The model under review builds one solid part; all positions refer to its coordinate system, in mm. Face numbers are marked on the shaded views. A direction names the side the tool comes from. Give positions to 0.01 mm unless a question says otherwise; leave off trailing zeros. Write each loop counter-clockwise with the first axis right and the second up, starting at its lowest first coordinate (ties: lowest second). Pieces come first, ordered by that corner, then holes. Notation, with made-up numbers: M -21.5,30.5 L 17.5,30.5 A25 cw 17.5,58.5 Z; hole C 35.25,-17 d11. An arc over 180 degrees is marked long. Write item = value, one per line. Start each with the question number.
```python
from build123d import *

# Parameters (mm, degrees)
F3_DEPTH = 25.4
F4_DEPTH = 25.4


with BuildPart() as f1:
    # F0 (on Front) → F1 (revolve)
    with BuildSketch(Plane.XZ):
        with BuildLine():
            Line((-95.25, -6.372012), (-95.25, -12.722012))
            Line((-95.25, -12.722012), (88.9, -12.722012))
            Line((88.9, -12.722012), (88.9, -0.022012))
            Line((88.9, -0.022012), (0, -0.022012))
            ThreePointArc((0, -0.022012), (-5.990472, -3.916067), (-12.7, -6.372012))
            Line((-12.7, -6.372012), (-45.3898, -6.372012))
            ThreePointArc((-45.3898, -6.372012), (-47.67075, -5.047272), (-47.6504, -2.409612))
            Line((-47.6504, -2.409612), (-52.4002, -2.409612))
            ThreePointArc((-52.4002, -2.409612), (-54.839819, -3.877688), (-57.640804, -4.389037))
            Line((-57.640804, -4.389037), (-93.039957, -4.389037))
            ThreePointArc((-93.039957, -4.389037), (-92.897345, -6.771022), (-95.25, -6.372012))
        make_face()
    revolve(axis=Axis((-3.175, 0, -12.722012), (1, 0, 0)))

    # F2 (on Front) → F3 (cut)
    with BuildSketch(Plane.XZ):
        with BuildLine():
            ThreePointArc((-12.482816, -6.482415), (1.656656, -10.036727), (16.186922, -11.232215))
            Line((16.186922, -11.232215), (87.516984, -11.232215))
            Line((87.516984, -11.232215), (89.117184, -12.832415))
            Line((89.117184, -12.832415), (96.563645, 18.124769))
            Line((96.563645, 18.124769), (7.196714, 21.508439))
            Line((7.196714, 21.508439), (-12.482816, -6.482415))
        make_face()
        with BuildLine():
            Line((96.563645, -43.789599), (89.117184, -12.832415))
            Line((89.117184, -12.832415), (87.516984, -14.432615))
            Line((87.516984, -14.432615), (16.186922, -14.432615))
            ThreePointArc((16.186922, -14.432615), (1.656656, -15.628103), (-12.482816, -19.182415))
            Line((-12.482816, -19.182415), (7.196714, -47.173269))
            Line((7.196714, -47.173269), (96.563645, -43.789599))
        make_face()
    extrude(amount=-F3_DEPTH, mode=Mode.SUBTRACT)

    # F2 (on Front) → F4 (cut)
    with BuildSketch(Plane.XZ):
        with BuildLine():
            ThreePointArc((-12.482816, -6.482415), (1.656656, -10.036727), (16.186922, -11.232215))
            Line((16.186922, -11.232215), (87.516984, -11.232215))
            Line((87.516984, -11.232215), (89.117184, -12.832415))
            Line((89.117184, -12.832415), (96.563645, 18.124769))
            Line((96.563645, 18.124769), (7.196714, 21.508439))
            Line((7.196714, 21.508439), (-12.482816, -6.482415))
        make_face()
        with BuildLine():
            Line((96.563645, -43.789599), (89.117184, -12.832415))
            Line((89.117184, -12.832415), (87.516984, -14.432615))
            Line((87.516984, -14.432615), (16.186922, -14.432615))
            ThreePointArc((16.186922, -14.432615), (1.656656, -15.628103), (-12.482816, -19.182415))
            Line((-12.482816, -19.182415), (7.196714, -47.173269))
            Line((7.196714, -47.173269), (96.563645, -43.789599))
        make_face()
    extrude(amount=F4_DEPTH, mode=Mode.SUBTRACT)


solid = f1.part
```
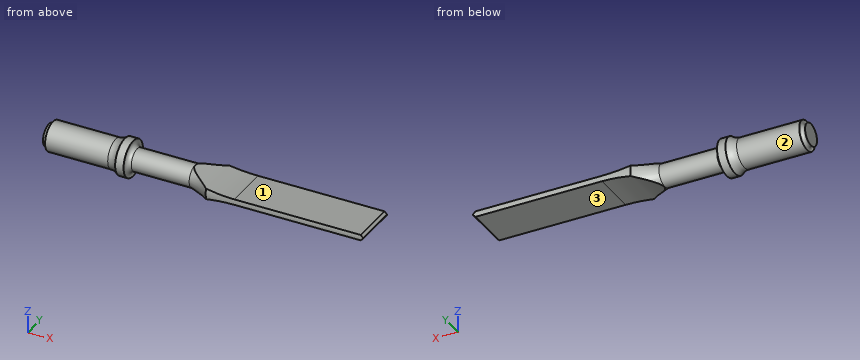
Item 1: Clearance check with flat-ended pins moving along their axes: P1, Ø2, axis at y = -4, z = -7, coming from the -X side; P2, Ø4, axis at x = -34, y = -1, coming from the -Z side; P3, Ø12.5, axis at x = 52.5, y = 0, coming from the +Z side; P4, Ø7.5, axis at x = 53.5, y = -3, coming from the -Z side. State where each tip first meets the part, or that it passes through.
Item 2: To check wall thickness, follow probe 1 along Z at (x, y) = (29.5, -7); probe 2 along Y at (x, z) = (-25, -12.5); probe 3 along Y at (x, z) = (-70, -12.25). State the ranges of each line that lie inside material, in increasing order. Write a range as [from, to].
Item 3: We need section C-C, the plane x = -3. Write out the cut boundary in (y, z), and give its area (3 significant figures).
Item 4: We need section B-B, the plane x = -69. Write out the cut boundary in (y, z), and give its area (3 significant figures).
Item 5: We need section A-A, the plane x = 40. Write out the cut boundary in (y, z).
Item 6: For the marked faces 1, 2 and 3, list the 3-axis set-ups (+Z, -Z, +X, -X, +Y, -Y) from which the entire face can be reached by the end or side of a thin tool; tool diameter is ignored.
Worked out:
q1.P1 = -95.25
q1.P2 = -19.07
q1.P3 = -11.23
q1.P4 = -14.43
q2.probe_1 = [-14.43, -11.23]
q2.probe_2 = [-6.35, 6.35]
q2.probe_3 = [-8.32, 8.32]
q3.outline = M -9.88,-9.14 A10.51 ccw -9.8,-16.53 L 9.8,-16.53 A10.51 ccw 9.88,-9.14 Z
q3.area = 152 mm²
q4.outline = C 0,-12.72 d16.67
q4.area = 218 mm²
q5.outline = M -12.61,-11.23 A12.7 ccw -12.58,-14.43 L 12.58,-14.43 A12.7 ccw 12.61,-11.23 Z
q6.face_1 = +Z, +X, +Y, -Y
q6.face_2 = -X
q6.face_3 = -Z, +X, +Y, -Y
